from build123d import *

# Parameters (mm, degrees)
SKETCH1_W           = 122.1
SKETCH1_H           = 197.8
BOSS_EXTRUDE2_DEPTH = 5
CUT_EXTRUDE1_DEPTH  = 5
SKETCH5_W           = 176.692600263
SKETCH5_H           = 67.834694549
CUT_EXTRUDE2_DEPTH  = 12
SKETCH6_W           = 148.50335492
SKETCH6_H           = 63.858757444
CUT_EXTRUDE3_DEPTH  = 19
SKETCH10_W          = 122.1
SKETCH10_H          = 5
BOSS_EXTRUDE4_DEPTH = 18.27


with BuildPart() as part:
    # Sketch1 → Boss-Extrude2 (new body)
    with BuildSketch(Plane(origin=(0, 0, 0), x_dir=(1, 0, 0), z_dir=(0, 1, 0))):
        with Locations((61.05, 98.9)):
            Rectangle(SKETCH1_W, SKETCH1_H)
    extrude(amount=BOSS_EXTRUDE2_DEPTH)

    # Sketch3 → Cut-Extrude1 (cut)
    with BuildSketch(Plane(origin=(0, 5, 0), x_dir=(1, 0, 0), z_dir=(0, 1, 0))):
        with BuildLine():
            Line((24.5, 152.22156802), (24.5, 45.30156802))
            ThreePointArc((24.5, 45.30156802), (17, 37.80156802), (9.5, 45.30156802))
            Line((9.5, 45.30156802), (9.5, 152.22156802))
            ThreePointArc((9.5, 152.22156802), (17, 159.72156802), (24.5, 152.22156802))
        make_face()
        with BuildLine():
            Line((97.6, 152.22156802), (97.6, 45.30156802))
            ThreePointArc((97.6, 45.30156802), (105.1, 37.80156802), (112.6, 45.30156802))
            Line((112.6, 45.30156802), (112.6, 152.22156802))
            ThreePointArc((112.6, 152.22156802), (105.1, 159.72156802), (97.6, 152.22156802))
        make_face()
    extrude(amount=-CUT_EXTRUDE1_DEPTH, mode=Mode.SUBTRACT)

    # Sketch5 → Cut-Extrude2 (cut)
    with BuildSketch(Plane(origin=(0, 0, -197.8), x_dir=(-1, 0, 0), z_dir=(0, 0, -1))):
        with Locations((-46.708276043, -7.602787765)):
            Rectangle(SKETCH5_W, SKETCH5_H)
    extrude(amount=-CUT_EXTRUDE2_DEPTH, mode=Mode.SUBTRACT)

    # Sketch6 → Cut-Extrude3 (cut)
    with BuildSketch(Plane.XY):
        with Locations((68.056552209, 0.930489014)):
            Rectangle(SKETCH6_W, SKETCH6_H)
    extrude(amount=-CUT_EXTRUDE3_DEPTH, mode=Mode.SUBTRACT)

    # Sketch10 → Boss-Extrude4 (add)
    with BuildSketch(Plane.XY.offset(-19)):
        with Locations((61.05, 2.5)):
            Rectangle(SKETCH10_W, SKETCH10_H)
    extrude(amount=BOSS_EXTRUDE4_DEPTH)


solid = part.part
Geometry check sheet. Reference: the model listing, model coordinates, mm. A direction names the side the tool comes from. Give positions to 0.01 mm unless a question says otherwise; leave off trailing zeros. Order: outer loops, then holes, each group sorted by start corner. A loop starts at its lowest first (then second) coordinate and runs counter-clockwise, first axis right, second up.
1) Tool access check on faces 4 (the flat face through (62, 3, -185.8)), 5 (the cylindrical face through (16.84, 2.54, -159.72)). Record the directions out of +Z, -Z, +X, -X, +Y, -Y that give a thin tool (end or side, any length) a straight path to the whole face; none if there is none.
Results are:
face 4: -Z, +X, -X, +Y, -Y
face 5: +Y, -Y
2) Material ranges on probe 1 along X at (y, z) = (2.65, -141.5); probe 2 along X at (y, z) = (2.2, -154.5); probe 3 along Z at (x, y) = (18.5, 2.25), recorded low to high.
Results are:
probe 1: x = 0 to 9.5, 24.5 to 97.6, 112.6 to 122.1
probe 2: x = 0 to 9.85, 24.15 to 97.95, 112.25 to 122.1
probe 3: z = -185.8 to -159.57, -37.95 to -0.73
3) Draft check along X on faces 1 (the flat face through (97.6, 3, -100)), 2 (the flat face through (0, 2, -95)), 3 (the flat face through (60, 0, -95)). Enter one of: released by +X, released by -X, zero draft, split by the parting line, or undercut.
Results are:
face 1: undercut
face 2: released by -X
face 3: zero draft
4) Cross-section at A-A (x = 17). Record the boundary of the cut face in (y, z), then the cut area to 3 significant figures.
Results are:
outline: (0, -185.8) - (5, -185.8) - (5, -159.72) - (0, -159.72) - close; (0, -37.8) - (5, -37.8) - (5, -0.73) - (0, -0.73) - close
area: 316 mm2
5) Cross-section at C-C (y = 1.25). Record the boundary of the cut face in (x, z).
Results are:
outline: (0, -185.8) - (122.1, -185.8) - (122.1, -0.73) - (0, -0.73) - close; hole (9.5, -152.22) arc R7.5 ccw to (24.5, -152.22) - (24.5, -45.3) arc R7.5 ccw to (9.5, -45.3) - close; hole (97.6, -152.22) arc R7.5 ccw to (112.6, -152.22) - (112.6, -45.3) arc R7.5 ccw to (97.6, -45.3) - close
6) Cross-section at B-B (z = -121). Record the boundary of the cut face in (x, y), then the cut area to 4 significant figures.
Results are:
outline: (0, 0) - (9.5, 0) - (9.5, 5) - (0, 5) - close; (24.5, 0) - (97.6, 0) - (97.6, 5) - (24.5, 5) - close; (112.6, 0) - (122.1, 0) - (122.1, 5) - (112.6, 5) - close
area: 460.5 mm2
